Answer from the drawing. Dimensions are ordinates in mm from the lowest x, y and z of the part. Give positions to 0.01 mm unless a question says otherwise; leave off trailing zeros. Loops run counter-clockwise (first coordinate to the right, second up) from the corner with the lowest first, then second, coordinate; pieces in that order, holes last.
Item 1: Consider line 1 along Y through (x, z) = (102, 2); line 2 along Y through (x, z) = (19.29, 0.6); line 3 along Y through (x, z) = (84, 1.4). Determine where each line is inside the solid, lowest interval first.
Item 2: Section A-A, the plane x = 136.5 is taken. Give the vertices of the cut face in (y, z), and give its area (3 significant figures).
Item 3: Section B-B, the plane x = 19.29 is taken. Give the vertices of the cut face in (y, z), and give its area (3 significant figures).
Item 4: Each of these flat-tipped pins is pushed along its axis until it touches: pin 1 Ø1 at (x, z) = (111, 1) entering from +Y (3 decimals); pin 2 Ø1.5 at (x, z) = (140, 1) entering from +Y. Where does it stop, or does it pass through?
Item 5: Section D-D, the plane z = 1.35 is taken. Give the number of separate pieces and of enclosed holes in the cut face, and give its area (3 significant figures).
Item 6: Section C-C, the plane y = 43 is taken. Give the vertices of the cut face in (x, z).
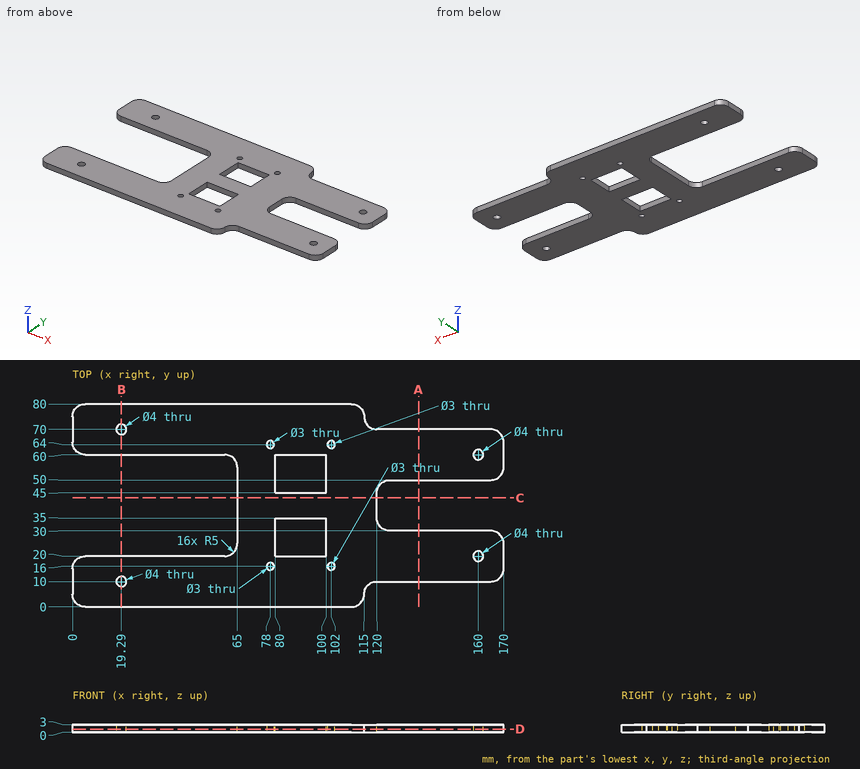
Worked answers:
1. line 1: y = 0 to 14.5, 17.5 to 62.5, 65.5 to 80
1. line 2: y = 0 to 8, 12 to 20, 60 to 68, 72 to 80
1. line 3: y = 0 to 20, 35 to 45, 60 to 80
2. outline: (10, 0) - (30, 0) - (30, 3) - (10, 3) - close; (50, 0) - (70, 0) - (70, 3) - (50, 3) - close
2. area: 120 mm2
3. outline: (0, 0) - (8, 0) - (8, 3) - (0, 3) - close; (12, 0) - (20, 0) - (20, 3) - (12, 3) - close; (60, 0) - (68, 0) - (68, 3) - (60, 3) - close; (72, 0) - (80, 0) - (80, 3) - (72, 3) - close
3. area: 96.0 mm2
4. pin 1: stops at y = 79.975
4. pin 2: stops at y = 70
5. separate pieces: 1
5. enclosed holes: 10
5. area: 8,200 mm2
6. outline: (65, 0) - (120, 0) - (120, 3) - (65, 3) - close
